from build123d import *

# Parameters (mm, degrees)
SKETCH1_R           = 34
BOSS_EXTRUDE1_DEPTH = 10
SKETCH2_R           = 32
BOSS_EXTRUDE2_DEPTH = 34
SKETCH3_R           = 26
CUT_EXTRUDE1_DEPTH  = 66.176682947
SKETCH4_W           = 27.053672336
SKETCH4_H           = 7.688048191
CUT_EXTRUDE2_DEPTH  = 34
CUT_EXTRUDE3_REACH  = 67.177
SKETCH5_W           = 49.442103022
SKETCH5_H           = 7.290390526


with BuildPart() as part:
    # Sketch1 → Boss-Extrude1 (new body)
    with BuildSketch(Plane(origin=(0, 0, 0), x_dir=(0, 0, -1), z_dir=(1, 0, 0))):
        Circle(SKETCH1_R)
    extrude(amount=BOSS_EXTRUDE1_DEPTH)

    # Sketch2 → Boss-Extrude2 (add)
    with BuildSketch(Plane(origin=(10, 0, 0), x_dir=(0, 0, -1), z_dir=(1, 0, 0))):
        Circle(SKETCH2_R)
    extrude(amount=BOSS_EXTRUDE2_DEPTH)

    # Sketch3 → Cut-Extrude1 (cut, through all)
    with BuildSketch(Plane(origin=(44, 0, 0), x_dir=(0, 0, -1), z_dir=(1, 0, 0))):
        Circle(SKETCH3_R)
    extrude(amount=-CUT_EXTRUDE1_DEPTH, mode=Mode.SUBTRACT)

    # Sketch4 → Cut-Extrude2 (cut)
    with BuildSketch(Plane(origin=(44, 0, 0), x_dir=(0, 0, -1), z_dir=(1, 0, 0))):
        with Locations((-0.035028199, 32.844024096)):
            Rectangle(SKETCH4_W, SKETCH4_H)
    extrude(amount=-CUT_EXTRUDE2_DEPTH, mode=Mode.SUBTRACT)

    # Sketch5 → Cut-Extrude3 (cut, up to next)
    with BuildSketch(Plane.ZY, mode=Mode.PRIVATE) as cut_extrude3_sk1:
        with Locations((1.06042044, 33.645195263)):
            Rectangle(SKETCH5_W, SKETCH5_H)
    cut_extrude3_tool1 = extrude(cut_extrude3_sk1.sketch, amount=-CUT_EXTRUDE3_REACH, mode=Mode.PRIVATE) & part.part
    add(cut_extrude3_tool1.solids().sort_by_distance((0, 33.645195, 1.06042))[0], mode=Mode.SUBTRACT)


solid = part.part
Design review of the part built by this model. Coordinates are the model's own, in mm. A direction names the side the tool comes from. Round coordinates to 2 decimals unless told otherwise and drop trailing zeros. Loops run counter-clockwise (first coordinate to the right, second up) from the corner with the lowest first, then second, coordinate; pieces in that order, holes last. Notation, with made-up numbers: (1.5, 30) - (20.5, 30) arc R38 ccw to (20.5, 68) - close; hole circle Ø7 at (73.5, 37). An arc over 180 degrees is marked (long way). One line per item, written item: value. Start each with the question number.
1) Draft analysis for pull direction Y (two halves, no side actions). For faces 1 (the flat face through (0, -26, 5)), 2 (the cylindrical face through (26.762, -31.978, 1.192)), 3 (the cylindrical face through (22.308, -15.821, 20.633)), state which applies: +Y half, -Y half, draft (parallel to the pull), parting line (faces both ways), or undercut.
2) Consider section A-A on z = 0. Give the boundary of the cut face in (x, y), then the cut area to 3 significant figures.
3) To check wall thickness, follow L1, parallel to Y at x = 25.5, z = 0; L2, parallel to Y at x = 5, z = 20; L3, parallel to Z at x = 4, y = 4.5. State the ranges of each line that lie inside material, in increasing order. Write a range as from..to.
4) Consider section D-D on z = -30. Give the boundary of the cut face in (x, y).
5) Insertion check: pin 1 Ø4 at (x, y) = (8.5, -6) entering from +Z; pin 2 Ø1.5 at (x, y) = (36, -12.5) entering from +Z; pin 3 Ø3 at (x, z) = (6, 4) entering from -Y. Each pin has a flat end and moves straight along its axis. Give the tip position at first contact, or say it passes through.
6) Consider section B-B on y = 0. Give the boundary of the cut face in (x, z).
7) For faces 4 (the flat face through (44, -26.2, 0.1)), 5 (the flat face through (10, -33, 0)), list the 3-axis set-ups (+Z, -Z, +X, -X, +Y, -Y) from which the entire face can be reached by the end or side of a thin tool; tool diameter is ignored.
Reported:
1. face 1: draft
1. face 2: parting line
1. face 3: undercut
2. outline: (0, -34) - (10, -34) - (10, -32) - (44, -32) - (44, -26) - (0, -26) - close; (0, 26) - (44, 26) - (44, 29) - (10, 29) - (10, 30) - (0, 30) - close
2. area: 426 mm^2
3. L1: y = -32..-26, 26..29
3. L2: y = -27.5..-16.61, 16.61..27.5
3. L3: z = -33.7..-25.61, 25.61..33.7
4. outline: (0, -16) - (10, -16) - (10, -11.14) - (44, -11.14) - (44, 11.14) - (10, 11.14) - (10, 16) - (0, 16) - close
5. pin 1: stops at z = 33.76
5. pin 2: stops at z = 29.76
5. pin 3: stops at y = -33.91
6. outline: (0, -34) - (10, -34) - (10, -32) - (44, -32) - (44, -26) - (0, -26) - close; (0, 26) - (44, 26) - (44, 32) - (10, 32) - (10, 34) - (0, 34) - close
7. face 4: +Z, -Z, +X, +Y, -Y
7. face 5: +X
